For this review, take the finished solid that the model builds, in its own axes (mm). Face numbers are marked on the shaded views. A direction names the side the tool comes from. Round coordinates to 2 decimals unless told otherwise and drop trailing zeros. Write each loop counter-clockwise with the first axis right and the second up, starting at its lowest first coordinate (ties: lowest second). Pieces come first, ordered by that corner, then holes. Notation, with made-up numbers: (61, 35.5) -> (114, 35.5) arc R17 cw to (114, 63.5) -> close; hole circle Ø10 at (-30, 67). An arc over 180 degrees is marked (long way). Write item = value, one per line. Start each with the question number.
```python
from build123d import *
from OCP.BRepFilletAPI import BRepFilletAPI_MakeChamfer

# Parameters (mm, degrees)
BOSS_EXTRUDE1_DEPTH = 4.5
BOSS_EXTRUDE2_DEPTH = 19
SKETCH4_W           = 6.6
SKETCH4_H           = 4.8
BOSS_EXTRUDE4_DEPTH = 2
SKETCH5_W           = 6.6
SKETCH5_H           = 2
CUT_EXTRUDE1_DEPTH  = 4.5
CUT_EXTRUDE2_REACH  = 45.186
CUT_EXTRUDE4_REACH  = 45.186
SKETCH9_W           = 6.6
SKETCH9_H           = 2
CUT_EXTRUDE5_DEPTH  = 16.8
FILLET3_R           = 3
SKETCH12_W          = 21.495
SKETCH12_H          = 5.5
CUT_EXTRUDE8_DEPTH  = 18
FILLET7_R           = 3
CHAMFER2_SIZE2      = 2
CHAMFER2_SIZE       = 4.5
CHAMFER3_SIZE       = 3.3
FILLET8_R           = 3.3
CHAMFER4_SIZE       = 9.5
CHAMFER4_SIZE_2     = 5.5


with BuildPart() as part:
    # Sketch1 → Boss-Extrude1 (new body)
    with BuildSketch(Plane(origin=(0, 0, 0), x_dir=(1, 0, 0), z_dir=(0, 1, 0))):
        with BuildLine():
            Line((-20.4975, -1.5), (-12.4975, -9.5))
            Line((-12.4975, -9.5), (12.4975, -9.5))
            Line((12.4975, -9.5), (20.4975, -1.5))
            ThreePointArc((20.4975, -1.5), (22.775674593, 4), (20.4975, 9.5))
            Line((20.4975, 9.5), (-20.4975, 9.5))
            ThreePointArc((-20.4975, 9.5), (-22.775674593, 4), (-20.4975, -1.5))
        make_face()
        with BuildLine():
            Line((-16.765266953, 5.767766953), (-16.033033906, 6.5))
            Line((-16.033033906, 6.5), (-13.961966094, 6.5))
            Line((-13.961966094, 6.5), (-13.229733047, 5.767766953))
            ThreePointArc((-13.229733047, 5.767766953), (-13.229733045, 2.232233049), (-16.765266949, 2.232233043))
            ThreePointArc((-16.765266949, 2.232233043), (-17.30719883, 3.043291416), (-17.4975, 4))
            ThreePointArc((-17.4975, 4), (-17.307198831, 4.956708581), (-16.765266953, 5.767766953))
        make_face(mode=Mode.SUBTRACT)
        with BuildLine():
            Line((13.229733047, 5.767766953), (13.961966094, 6.5))
            Line((13.961966094, 6.5), (16.033033906, 6.5))
            Line((16.033033906, 6.5), (16.765266953, 5.767766953))
            ThreePointArc((16.765266953, 5.767766953), (16.765266949, 2.232233043), (13.229733038, 2.232233056))
            ThreePointArc((13.229733038, 2.232233056), (12.4975, 4.000000006), (13.229733047, 5.767766953))
        make_face(mode=Mode.SUBTRACT)
    extrude(amount=BOSS_EXTRUDE1_DEPTH)

    # Sketch2 → Boss-Extrude2 (add, through all)
    with BuildSketch(Plane(origin=(0, 0, -9.5), x_dir=(-1, 0, 0), z_dir=(0, 0, -1))):
        Polygon((-7.3, 4.5), (-3.3, 4.5), (-3.3, 27.5), (3.3, 27.5), (3.3, 4.5), (7.3, 4.5), (7.3, 29.5), (-7.3, 29.5), align=None)
    extrude(amount=-BOSS_EXTRUDE2_DEPTH)

    # Sketch4 → Boss-Extrude4 (add)
    with BuildSketch(Plane(origin=(0, 4.5, 0), x_dir=(1, 0, 0), z_dir=(0, 1, 0))):
        with Locations((0, 7.1)):
            Rectangle(SKETCH4_W, SKETCH4_H)
    extrude(amount=BOSS_EXTRUDE4_DEPTH)

    # Sketch5 → Cut-Extrude1 (cut)
    with BuildSketch(Plane.XY.offset(9.5)):
        with Locations((0, 3.5)):
            Rectangle(SKETCH5_W, SKETCH5_H)
    extrude(amount=-CUT_EXTRUDE1_DEPTH, mode=Mode.SUBTRACT)

    # Sketch6 → Cut-Extrude2 (cut, up to next)
    with BuildSketch(Plane(origin=(7.3, 0, 0), x_dir=(0, 0, -1), z_dir=(1, 0, 0)), mode=Mode.PRIVATE) as cut_extrude2_sk1:
        with BuildLine():
            Line((-1.65, 20.059188309), (-2.045405845, 20.454594155))
            ThreePointArc((-2.045405845, 20.454594155), (-4.35, 19.5), (-2.045405845, 18.545405845))
            Line((-2.045405845, 18.545405845), (-1.65, 18.940811691))
            Line((-1.65, 18.940811691), (-1.65, 20.059188309))
        make_face()
    cut_extrude2_tool1 = extrude(cut_extrude2_sk1.sketch, amount=-CUT_EXTRUDE2_REACH, mode=Mode.PRIVATE) & part.part
    # Sketch6 → Cut-Extrude2 (cut, up to next)
    with BuildSketch(Plane(origin=(7.3, 0, 0), x_dir=(0, 0, -1), z_dir=(1, 0, 0)), mode=Mode.PRIVATE) as cut_extrude2_sk2:
        with BuildLine():
            Line((-1.65, 10.059188309), (-2.045405845, 10.454594155))
            ThreePointArc((-2.045405845, 10.454594155), (-4.35, 9.5), (-2.045405845, 8.545405845))
            Line((-2.045405845, 8.545405845), (-1.65, 8.940811691))
            Line((-1.65, 8.940811691), (-1.65, 10.059188309))
        make_face()
    cut_extrude2_tool2 = extrude(cut_extrude2_sk2.sketch, amount=-CUT_EXTRUDE2_REACH, mode=Mode.PRIVATE) & part.part
    add(cut_extrude2_tool1.solids().sort_by_distance((7.3, 19.5, 2.982857))[0], mode=Mode.SUBTRACT)
    add(cut_extrude2_tool2.solids().sort_by_distance((7.3, 9.5, 2.982857))[0], mode=Mode.SUBTRACT)

    # Sketch8 → Cut-Extrude4 (cut, up to next)
    with BuildSketch(Plane.ZY.offset(7.3), mode=Mode.PRIVATE) as cut_extrude4_sk1:
        with BuildLine():
            Line((1.25, 10.224873734), (1.25, 8.775126266))
            Line((1.25, 8.775126266), (1.762563133, 8.262563133))
            ThreePointArc((1.762563133, 8.262563133), (4.75, 9.5), (1.762563133, 10.737436867))
            Line((1.762563133, 10.737436867), (1.25, 10.224873734))
        make_face()
    cut_extrude4_tool1 = extrude(cut_extrude4_sk1.sketch, amount=-CUT_EXTRUDE4_REACH, mode=Mode.PRIVATE) & part.part
    # Sketch8 → Cut-Extrude4 (cut, up to next)
    with BuildSketch(Plane.ZY.offset(7.3), mode=Mode.PRIVATE) as cut_extrude4_sk2:
        with BuildLine():
            Line((1.25, 20.224873734), (1.25, 18.775126266))
            Line((1.25, 18.775126266), (1.762563133, 18.262563133))
            ThreePointArc((1.762563133, 18.262563133), (4.75, 19.5), (1.762563133, 20.737436867))
            Line((1.762563133, 20.737436867), (1.25, 20.224873734))
        make_face()
    cut_extrude4_tool2 = extrude(cut_extrude4_sk2.sketch, amount=-CUT_EXTRUDE4_REACH, mode=Mode.PRIVATE) & part.part
    add(cut_extrude4_tool1.solids().sort_by_distance((-7.3, 9.5, 2.977778))[0], mode=Mode.SUBTRACT)
    add(cut_extrude4_tool2.solids().sort_by_distance((-7.3, 19.5, 2.977778))[0], mode=Mode.SUBTRACT)

    # Sketch9 → Cut-Extrude5 (cut)
    with BuildSketch(Plane.XY.offset(9.5)):
        with Locations((0, 28.5)):
            Rectangle(SKETCH9_W, SKETCH9_H)
    extrude(amount=-CUT_EXTRUDE5_DEPTH, mode=Mode.SUBTRACT)

    # Fillet3
    fillet3_edges = [part.edges().sort_by_distance(p)[0] for p in [
        (-7.3, 4.5, 0),
        (7.3, 4.5, 0),
    ]]
    fillet(fillet3_edges, radius=FILLET3_R)

    # Sketch12 → Cut-Extrude8 (cut)
    with BuildSketch(Plane.XZ):
        with Locations((0, -6.75)):
            Rectangle(SKETCH12_W, SKETCH12_H)
    extrude(amount=-CUT_EXTRUDE8_DEPTH, mode=Mode.SUBTRACT)

    # Fillet7
    fillet7_edges = [part.edges().sort_by_distance(p)[0] for p in [
        (-7.3, 29.5, 0),
        (7.3, 29.5, 0),
    ]]
    fillet(fillet7_edges, radius=FILLET7_R)

    # Chamfer2
    chamfer2_edges = [part.edges().sort_by_distance(p)[0] for p in [
        (0, 2.5, 5),
    ]]
    chamfer2_side = [part.faces().sort_by_distance(p)[0] for p in [
        (0, 2.5, 5.04),
    ]]
    chamfer(chamfer2_edges, length=CHAMFER2_SIZE - 0.0001, length2=CHAMFER2_SIZE2 - 0.0001, reference=chamfer2_side[0])  # a hair under: the kernel refuses the full size

    # Chamfer3
    chamfer3_edges = [part.edges().sort_by_distance(p)[0] for p in [
        (-3.3, 28.5, -7.3),
        (3.3, 28.5, -7.3),
    ]]
    chamfer(chamfer3_edges, length=CHAMFER3_SIZE - 0.0001)  # a hair under: the kernel refuses the full size

    # Fillet8
    fillet8_edges = [part.edges().sort_by_distance(p)[0] for p in [
        (-3.3, 28.5, -4.0001),
        (3.3, 28.5, -4.0001),
    ]]
    fillet(fillet8_edges, radius=FILLET8_R)

    # Chamfer4
    chamfer4_edges_1 = [part.edges().sort_by_distance(p)[0] for p in [
        (-5.3, 18, -9.5),
    ]]
    chamfer4_side_1 = [part.faces().sort_by_distance(p)[0] for p in [
        (-5.3, 18.11, -9.5),
    ]]
    chamfer4_edges_2 = [part.edges().sort_by_distance(p)[0] for p in [
        (5.3, 18, -9.5),
    ]]
    chamfer4_side_2 = [part.faces().sort_by_distance(p)[0] for p in [
        (5.3, 18, -9.39),
    ]]
    chamfer4 = BRepFilletAPI_MakeChamfer(part.part.solid().wrapped)
    for e in chamfer4_edges_1:
        chamfer4.Add(CHAMFER4_SIZE - 0.0001, CHAMFER4_SIZE_2 - 0.0001, e.wrapped, chamfer4_side_1[0].wrapped)
    for e in chamfer4_edges_2:
        chamfer4.Add(CHAMFER4_SIZE_2 - 0.0001, CHAMFER4_SIZE - 0.0001, e.wrapped, chamfer4_side_2[0].wrapped)
    add(Compound.cast(chamfer4.Shape()), mode=Mode.REPLACE)  # a hair under: the kernel refuses the full size


solid = part.part
```
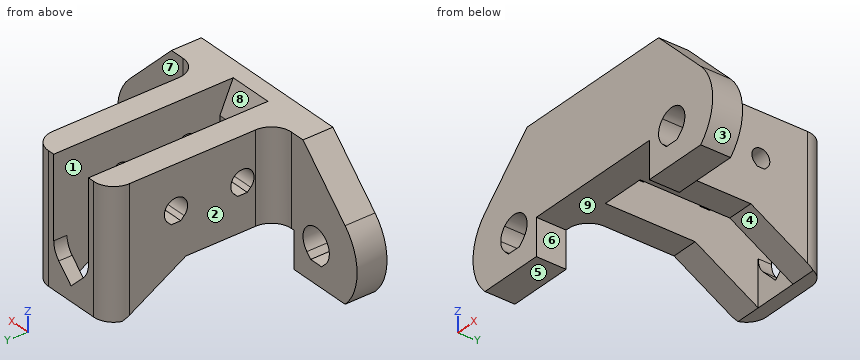
1. Machinability: for the marked faces 5, 6, 7, 8 and 9, which of the approach directions +Z, -Z, +X, -X, +Y, -Y give a long, thin tool a straight path to every point of the face, cutting with its end or side? Answer none if there is none.
2. Consider section B-B, the plane z = 3. Give the number of separate pieces and of enclosed holes in the cut face, then the cut area to 3 significant figures.
3. Draft analysis for pull direction X (two halves, no side actions). For the marked faces 1, 2, 3 and 4, state which applies: +X half, -X half, draft (parallel to the pull), parting line (faces both ways), or undercut.
4. Consider section A-A, the plane y = 12.5. Give the boundary of the cut face in (x, z).
5. Clearance check with flat-ended pins moving along their axes: pin 1 Ø12 at (x, y) = (-4, 11) entering from -Z; pin 2 Ø6 at (x, z) = (-9.5, -7.5) entering from +Y; pin 3 Ø8 at (y, z) = (15.5, 6) entering from +X. State where each tip first meets the part, or that it passes through.
6. Wall thickness on L1, parallel to X at y = 17.5, z = -0.25; L2, parallel to Y at x = -5.3, z = 3; L3, parallel to Y at x = 16.5, z = -6.75: over which ranges is each line inside the solid? List them lowest first. Write a range as from..to.
7. Consider section D-D, the plane y = 19.5. Give the boundary of the cut face in (x, z), then the cut area to 3 significant figures.
Outcome:
q1.face_5 = -Z, +X, -X, +Y, -Y
q1.face_6 = -Z, +Y, -Y
q1.face_7 = +Z, -Z, +X, +Y
q1.face_8 = +Z, +Y
q1.face_9 = -Z, -Y
q2.separate_pieces = 5
q2.enclosed_holes = 0
q2.area = 321 mm2
q3.face_1 = undercut
q3.face_2 = -X half
q3.face_3 = +X half
q3.face_4 = draft
q4.outline = (-7.3, -4) -> (-3.3, -4) -> (-3.3, 9.5) -> (-7.3, 9.5) -> close; (3.3, -4) -> (7.3, -4) -> (7.3, 9.5) -> (3.3, 9.5) -> close
q5.pin_1 = -4
q5.pin_2 = 28.54
q5.pin_3 = 7.3
q6.L1 = -7.3..-3.3, 3.3..7.3
q6.L2 = 0..7.75, 11.25..17.75, 21.25..29.33
q6.L3 = 0..4.5
q7.outline = (-7.3, -4.87) -> (-3.3, -4.87) -> (-3.3, 1.25) -> (-7.3, 1.25) -> close; (-7.3, 4.75) -> (-3.3, 4.75) -> (-3.3, 9.5) -> (-7.3, 9.5) -> close; (3.3, -4.87) -> (7.3, -4.87) -> (7.3, 1.65) -> (3.3, 1.65) -> close; (3.3, 4.35) -> (7.3, 4.35) -> (7.3, 9.5) -> (3.3, 9.5) -> close
q7.area = 90.1 mm2
